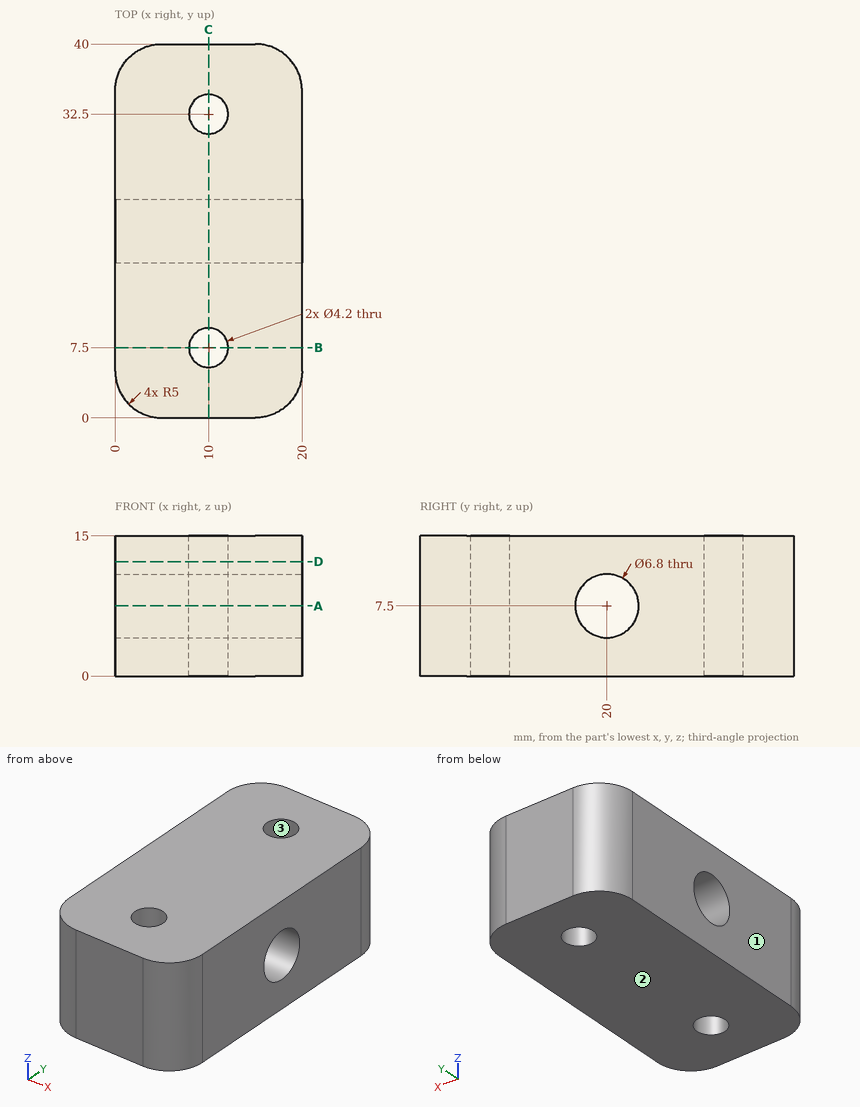
The figure shows three views and two pictorial views of one solid part (mm, origin at its lowest corner). Answer the questions. Give positions to 0.01 mm unless a question says otherwise; leave off trailing zeros. Order: outer loops, then holes, each group sorted by start corner. A loop starts at its lowest first (then second) coordinate and runs counter-clockwise, first axis right, second up. Notation, with made-up numbers: (36.25, 22) -> (83.25, 22) arc R32 cw to (83.25, 53) -> close; hole circle Ø8 at (24, 84). An arc over 180 degrees is marked (long way). Answer as CSV lines item,"result". Start each with the question number.
Q1. Given pin 1 (10 mm diameter, centred on x = 8.5, y = 21.5, fed in from -Z); pin 2 (3 mm diameter, centred on x = 3, z = 10, fed in from -Y); pin 3 (1 mm diameter, centred on x = 10.5, y = 33.5, fed in from -Z), each flat-ended and moving along its own axis, determine where each tip first touches the part or whether it passes through.
Q2. A cutting plane is placed at B-B (y = 7.5). Determine the outline of the cut face in (x, z), then the cut area to 3 significant figures.
Q3. Determine the mould class of the marked faces 1, 2 and 3 for opening direction X: pulls with the +X half, pulls with the -X half, needs draft (parallel to the pull), parting line crosses it, or undercut.
Q4. A cutting plane is placed at C-C (x = 10). Determine the outline of the cut face in (y, z), then the cut area to 3 significant figures.
Q5. Find the intervals of material crossed by L1, parallel to Y at x = 15, z = 7.5; L2, parallel to Y at x = 10.5, z = 8; L3, parallel to Y at x = 11.5, z = 3.75, in increasing order.
Q6. A cutting plane is placed at D-D (z = 12.25). Determine the outline of the cut face in (x, y), then the cut area to 3 significant figures.
Q7. A cutting plane is placed at A-A (z = 7.5). Determine the outline of the cut face in (x, y).
Results found:
1,pin 1,"z = 0"
1,pin 2,"y = 0.03"
1,pin 3,"through"
2,outline,"(0, 0) -> (7.9, 0) -> (7.9, 15) -> (0, 15) -> close; (12.1, 0) -> (20, 0) -> (20, 15) -> (12.1, 15) -> close"
2,area,"237 mm2"
3,face 1,"pulls with the -X half"
3,face 2,"needs draft"
3,face 3,"undercut"
4,outline,"(0, 0) -> (5.4, 0) -> (5.4, 15) -> (0, 15) -> close; (9.6, 0) -> (30.4, 0) -> (30.4, 15) -> (9.6, 15) -> close; (34.6, 0) -> (40, 0) -> (40, 15) -> (34.6, 15) -> close; hole circle Ø6.8 at (20, 7.5)"
4,area,"438 mm2"
5,L1,"0 to 16.6, 23.4 to 40"
5,L2,"0 to 5.46, 9.54 to 16.64, 23.36 to 30.46, 34.54 to 40"
5,L3,"0 to 6.03, 8.97 to 31.03, 33.97 to 40"
6,outline,"(0, 5) arc R5 ccw to (5, 0) -> (15, 0) arc R5 ccw to (20, 5) -> (20, 35) arc R5 ccw to (15, 40) -> (5, 40) arc R5 ccw to (0, 35) -> close; hole circle Ø4.2 at (10, 7.5); hole circle Ø4.2 at (10, 32.5)"
6,area,"751 mm2"
7,outline,"(0, 5) arc R5 ccw to (5, 0) -> (15, 0) arc R5 ccw to (20, 5) -> (20, 16.6) -> (0, 16.6) -> close; (0, 23.4) -> (20, 23.4) -> (20, 35) arc R5 ccw to (15, 40) -> (5, 40) arc R5 ccw to (0, 35) -> close; hole circle Ø4.2 at (10, 7.5); hole circle Ø4.2 at (10, 32.5)"
